Here's how the part is built. I have some questions about the finished solid (model axes, mm). A direction names the side the tool comes from. Round coordinates to 2 decimals unless told otherwise and drop trailing zeros. Write each loop counter-clockwise with the first axis right and the second up, starting at its lowest first coordinate (ties: lowest second). Pieces come first, ordered by that corner, then holes. Notation, with made-up numbers: M 58.25,-4.5 L 65.25,-4.5 A16 cw 65.25,25.5 Z; hole C 54,25 d4. An arc over 180 degrees is marked long. Use one line per item in the form item = value. Start each with the question number.
Q1. For faces 1 (the face through (-5, 11, -3132.136)), 2 (the face through (-20.744, 16.435, -3138.929)), which set-ups out of +Z, -Z, +X, -X, +Y, -Y let a thin tool reach every point of the face, with its end or its side?
Q2. I need wall thicknesses on line 1 along Z through (x, y) = (-13, 5.5); line 2 along X through (y, z) = (1.5, -3133.5). Which ranges of each line are inside material? Lowest first, please. Write a range as from..to.
Q3. I want a section at A-A on x = 0. List the corners of the cut face in (y, z) for me (3 decimals), and give its area (3 significant figures).
Q4. We'd pull the mould along Y, two halves only. Please class faces 3 (the face through (9.396, 11, -3131)), 4 (the face through (-19.34, 0, -3145.94)), 5 (the face through (-20.744, 5.162, -3150.604)), 6 (the face through (-19.34, 22.225, -3145.94)): +Y half, -Y half, draft (parallel to the pull), parting line (faces both ways), or undercut.
Q5. I want a section at C-C on y = 12.75. List the corners of the cut face in (x, z) for me.
Q6. I want a section at B-B on y = 5.08. State how many separate pieces and enclosed holes the cut face has, and give its area (3 significant figures).
Q7. I'm going to push flat-ended pins straight in: pin 1 Ø8 at (y, z) = (11, -3140.5) entering from +X; pin 2 Ø3.5 at (x, y) = (-10.92, 17.14) entering from -Z. Where does each tip first touch, or does it pass through?
Q8. I want a section at D-D on z = -3155. List the corners of the cut face in (x, y) for me (3 decimals), and give its area (3 significant figures).
Autodesk Inventor part; units mm, degrees
ref_plane "YZ Plane" through (0, 0, 0) normal (1, 0, 0) x (0, 1, 0)
ref_plane "XZ Plane" through (0, 0, 0) normal (0, 1, 0) x (-1, 0, 0)
ref_plane "XY Plane" through (0, 0, 0) normal (0, 0, 1) x (1, 0, 0)
sketch "Sketch1" plane through (0, 0, 0) normal (0, 1, 0) x (-1, 0, 0)
  line L0 (22.3541, -3128.9614) -> (-9.3959, -3128.9614)
  line L1 (-9.3959, -3128.9614) -> (-9.3959, -3132.1364)
  line L2 (-9.3959, -3132.1364) -> (22.3541, -3132.1364)
  line L3 (22.3541, -3132.1364) -> (22.3541, -3128.9614)
  line L4 (22.3541, -3128.9614) -> (19.1791, -3128.9614)
  line L5 (19.1791, -3128.9614) -> (19.1791, -3157.5364)
  line L6 (19.1791, -3157.5364) -> (22.3541, -3157.5364)
  line L7 (22.3541, -3157.5364) -> (22.3541, -3128.9614)
  line L8 (22.3541, -3157.5364) -> (-9.3959, -3157.5364)
  line L9 (-9.3959, -3157.5364) -> (-9.3959, -3160.7114)
  line L10 (-9.3959, -3160.7114) -> (22.3541, -3160.7114)
  line L11 (22.3541, -3160.7114) -> (22.3541, -3157.5364)
  point P0 (0, 0)
  point P1 (19.1791, -3132.1364)
  dimension "d0" = 31.75
  dimension "d1" = 3.175
  dimension "d2" = 3.175
  dimension "d4" = 31.75
  dimension "d5" = 3.175
  dimension "d22" = 31.75
extrude "Extrusion1" add sketch "Sketch1" along normal blind 22.225
sketch "Sketch2" plane through (-19.1791, 0, -3132.1364) normal (1, 0, 0) x (0, 0, -1)
  line L0 (-3.175, 0) -> (0, 0)
  line L1 (0, 0) -> (0, 22.225)
  line L2 (-3.175, 22.225) -> (0, 22.225)
  line L3 (-3.175, 0) -> (-3.175, 22.225)
  line L4 (25.4, 0) -> (28.575, 0)
  line L5 (28.575, 0) -> (28.575, 22.225)
  line L6 (25.4, 22.225) -> (28.575, 22.225)
  line L7 (25.4, 0) -> (25.4, 22.225)
  circle A0 centre (5.08, 17.145) radius 1.8542
  circle A1 centre (20.32, 17.145) radius 1.8542
  circle A2 centre (5.08, 5.08) radius 1.8542
  circle A3 centre (20.32, 5.08) radius 1.8542
  line L8 (0, 22.225) -> (25.4, 22.225)
  line L9 (0, 0) -> (25.4, 0)
  point P0 (-3132.1364, 0)
  dimension "d8" = 3.7084
  dimension "d9" = 3.7084
  dimension "d10" = 3.7084
  dimension "d11" = 3.7084
  dimension "d12" = 5.08
  dimension "d13" = 5.08
  dimension "d14" = 5.08
  dimension "d15" = 5.08
  dimension "d16" = 5.08
  dimension "d17" = 5.08
  dimension "d18" = 5.08
  dimension "d19" = 5.08
extrude "Extrusion2" cut sketch "Sketch2" against normal blind 25.4 contours A0 | A1 | A2 | A3
sketch "Sketch3" plane through (-22.3541, 0, -3128.9614) normal (0, 0, 1) x (1, 0, 0)
  circle A0 centre (26.67, 17.145) radius 1.8542
  circle A1 centre (11.43, 17.145) radius 1.8542
  circle A2 centre (26.67, 5.08) radius 1.8542
  circle A3 centre (11.43, 5.08) radius 1.8542
  line L0 (0, 0) -> (31.75, 0)
  line L1 (31.75, 0) -> (31.75, 22.225)
  line L2 (0, 22.225) -> (31.75, 22.225)
  line L3 (0, 0) -> (0, 22.225)
  point P0 (22.3541, 0)
  dimension "d23" = 3.7084
  dimension "d24" = 3.7084
  dimension "d25" = 3.7084
  dimension "d26" = 3.7084
  dimension "d27" = 5.08
  dimension "d28" = 5.08
  dimension "d29" = 11.43
  dimension "d30" = 11.43
  dimension "d31" = 5.08
  dimension "d32" = 5.08
  dimension "d33" = 5.08
  dimension "d34" = 5.08
extrude "Extrusion3" cut sketch "Sketch3" against normal blind 50.8 contours A0 | A1 | A2 | A3
equation "\"d4\" = d0"
equation "\"d13\" = d12"
equation "\"d14\" = d12"
equation "\"d15\" = d12"
equation "\"d17\" = d16"
equation "\"d18\" = d16"
equation "\"d19\" = d16"
equation "\"d28\" = d27"
equation "\"d30\" = d29"
equation "\"d32\" = d31"
equation "\"d33\" = d31"
equation "\"d34\" = d31"
properties part number "connector"
Reported:
q1.face_1 = +X, +Y, -Y
q1.face_2 = +X, -X
q2.line_1 = -3160.71..-3157.54, -3132.14..-3128.96
q2.line_2 = -22.35..-19.18
q3.outline = M 0,-3160.711 L 22.225,-3160.711 L 22.225,-3157.536 L 0,-3157.536 Z; M 0,-3132.136 L 22.225,-3132.136 L 22.225,-3128.961 L 0,-3128.961 Z
q3.area = 141 mm^2
q4.face_3 = draft
q4.face_4 = -Y half
q4.face_5 = undercut
q4.face_6 = +Y half
q5.outline = M -22.35,-3160.71 L 9.4,-3160.71 L 9.4,-3157.54 L -19.18,-3157.54 L -19.18,-3132.14 L 9.4,-3132.14 L 9.4,-3128.96 L -22.35,-3128.96 Z
q6.separate_pieces = 7
q6.enclosed_holes = 0
q6.area = 212 mm^2
q7.pin_1 = -19.18
q7.pin_2 = through
q8.outline = M -22.354,0 L -19.179,0 L -19.179,22.225 L -22.354,22.225 Z
q8.area = 70.6 mm^2
